Check sheet for the modelled part. Datum: model origin and axes. Units: mm. A direction names the side the tool comes from. Round coordinates to 2 decimals unless told otherwise and drop trailing zeros. Loops run counter-clockwise (first coordinate to the right, second up) from the corner with the lowest first, then second, coordinate; pieces in that order, holes last. Notation, with made-up numbers: (-21.75, 71) -> (33.25, 71) arc R13 ccw to (33.25, 85) -> close; hole circle Ø3 at (1, -2). An arc over 180 degrees is marked (long way). Return JSON: item names as keys, results as strings.
from build123d import *

# Parameters (mm, degrees)
ESQUISSE3_R             = 35
BOSS_EXTRU_3_DEPTH      = 5
ESQUISSE4_W             = 45
ESQUISSE4_H             = 30
ENL_V_MAT_EXTRU_1_DEPTH = 161.669919512


with BuildPart() as part:
    # Esquisse3 → Boss.-Extru.3 (new body)
    with BuildSketch(Plane(origin=(0, 0, 0), x_dir=(1, 0, 0), z_dir=(0, 1, 0))):
        with BuildLine():
            Line((-115, -25), (-25, -25))
            Line((-25, -25), (-24.99494949, -24.500051021))
            ThreePointArc((-24.99494949, -24.500051021), (-34.998214236, 0.353553761), (-24.494897428, 25))
            Line((-24.494897428, 25), (-25, 25))
            Line((-25, 25), (-115, 25))
            Line((-115, 25), (-115, -25))
        make_face()
        Circle(ESQUISSE3_R)
        Polygon((-9.403186381, -33.713203436), (35.849364905, -112.092921435), (79.150635095, -87.092921435), (34.150635095, -9.150635095), align=None)
        with BuildLine():
            Line((-24.494897428, 25), (-24.99494949, -24.500051021))
            ThreePointArc((-24.99494949, -24.500051021), (-17.805293657, -30.132565736), (-9.403186381, -33.713203436))
            Line((-9.403186381, -33.713203436), (33.715141323, -9.396235714))
            ThreePointArc((33.715141323, -9.396235714), (34.677297662, -4.741837919), (35, 0))
            ThreePointArc((35, 0), (34.72342821, 4.391302011), (33.898083809, 8.713203436))
            Line((33.898083809, 8.713203436), (-8.720191833, 33.896286735))
            ThreePointArc((-8.720191833, 33.896286735), (-17.19292058, 30.486119496), (-24.494897428, 25))
        make_face()
        Circle(ESQUISSE3_R)
        Polygon((33.898083809, 8.713203436), (79.150635095, 87.092921435), (35.849364905, 112.092921435), (-9.150635095, 34.150635095), align=None)
        with BuildLine():
            ThreePointArc((33.898083809, 8.713203436), (17.805293657, 30.132565736), (-8.720191833, 33.896286735))
            Line((-8.720191833, 33.896286735), (33.898083809, 8.713203436))
        make_face()
    extrude(amount=BOSS_EXTRU_3_DEPTH)

    # Esquisse4 → Enlèv. mat.-Extru.1 (cut, through all)
    with BuildSketch(Plane(origin=(0, 5, 0), x_dir=(1, 0, 0), z_dir=(0, 1, 0))):
        Rectangle(ESQUISSE4_W, ESQUISSE4_H)
    extrude(amount=-ENL_V_MAT_EXTRU_1_DEPTH, mode=Mode.SUBTRACT)


solid = part.part
Q1. Section check C-C (x = -65). Record the boundary of the cut face in (y, z), then the cut area to 3 significant figures.
Results list:
{"outline": "(0, -25) -> (5, -25) -> (5, 25) -> (0, 25) -> close", "area": "250 mm^2"}
Q2. Draft check along Z on faces 1 (the flat face through (-22.5, 3, 0)), 2 (the flat face through (22.5, 3, 0)), 3 (the flat face through (-69, 2, -25)), 4 (the flat face through (-4, 5, -17)). Enter one of: released by +Z, released by -Z, zero draft, split by the parting line, or undercut.
Results list:
{"face 1": "undercut", "face 2": "undercut", "face 3": "released by -Z", "face 4": "zero draft"}
Q3. Section check B-B (x = 38.5). Record the boundary of the cut face in (y, z), then the cut area to 3 significant figures.
Results list:
{"outline": "(0, -110.56) -> (5, -110.56) -> (5, -16.68) -> (0, -16.68) -> close; (0, 16.68) -> (5, 16.68) -> (5, 110.56) -> (0, 110.56) -> close", "area": "939 mm^2"}
Q4. Section check D-D (z = 72). Record the boundary of the cut face in (x, y), then the cut area to 3 significant figures.
Results list:
{"outline": "(12.7, 0) -> (70.44, 0) -> (70.44, 5) -> (12.7, 5) -> close", "area": "289 mm^2"}
Q5. Tool access check on faces 5 (the flat face through (0, 3, -15)), 6 (the flat face through (56.208, 2.465, -47.354)), 7 (the flat face through (-4, 0, -17)), 8 (the flat face through (-71, 2, 25)). Record the directions out of +Z, -Z, +X, -X, +Y, -Y that give a thin tool (end or side, any length) a straight path to the whole face; none if there is none.
Results list:
{"face 5": "+Y, -Y", "face 6": "+X, +Y, -Y", "face 7": "+Z, -Z, +X, -X, -Y", "face 8": "+Z, -X, +Y, -Y"}
Q6. Material ranges on line 1 (Z direction, x = -89, y = 3.35); line 2 (Z direction, x = 5.5, y = 1.25); line 3 (Z direction, x = 41, y = 0.8), recorded low to high.
Results list:
{"line 1": "-25 to 25", "line 2": "-59.53 to -15, 15 to 59.53", "line 3": "-109.12 to -21.01, 21.01 to 109.12"}
Q7. Section check A-A (y = 1.45). Record the boundary of the cut face in (x, z).
Results list:
{"outline": "(-115, -25) -> (-24.49, -25) arc R35 ccw to (-8.72, -33.9) -> (-9.15, -34.15) -> (35.85, -112.09) -> (79.15, -87.09) -> (33.9, -8.71) arc R35 ccw to (33.72, 9.4) -> (34.15, 9.15) -> (79.15, 87.09) -> (35.85, 112.09) -> (-9.4, 33.71) arc R35 ccw to (-24.99, 24.5) -> (-25, 25) -> (-115, 25) -> close; hole (-22.5, -15) -> (22.5, -15) -> (22.5, 15) -> (-22.5, 15) -> close"}
Q8. Go/stop test with flat-tipped pins: pin 1 (2 mm diameter, centred on y = 2.5, z = -50.5, fed in from -X); pin 2 (1.5 mm diameter, centred on x = -4.5, y = 3.5, fed in from -Z); pin 3 (1 mm diameter, centred on y = 3, z = 7, fed in from +X). Record where each tip stops, or that it passes through.
Results list:
{"pin 1": "x = -0.29", "pin 2": "z = -43.5", "pin 3": "x = 34.39"}
